Study the drawing (mm; zero at the part's minimum x, y, z) and answer. Give positions to 0.01 mm unless a question says otherwise; leave off trailing zeros. Write each loop counter-clockwise with the first axis right and the second up, starting at its lowest first coordinate (ties: lowest second). Pieces come first, ordered by that corner, then holes. Notation, with made-up numbers: (7, 18.5) - (22, 18.5) arc R12 cw to (22, 29.5) - close; hole circle Ø11 at (0, -3.5). An arc over 180 degrees is marked (long way). Answer in a Markdown table with one row per item. Add a question column.
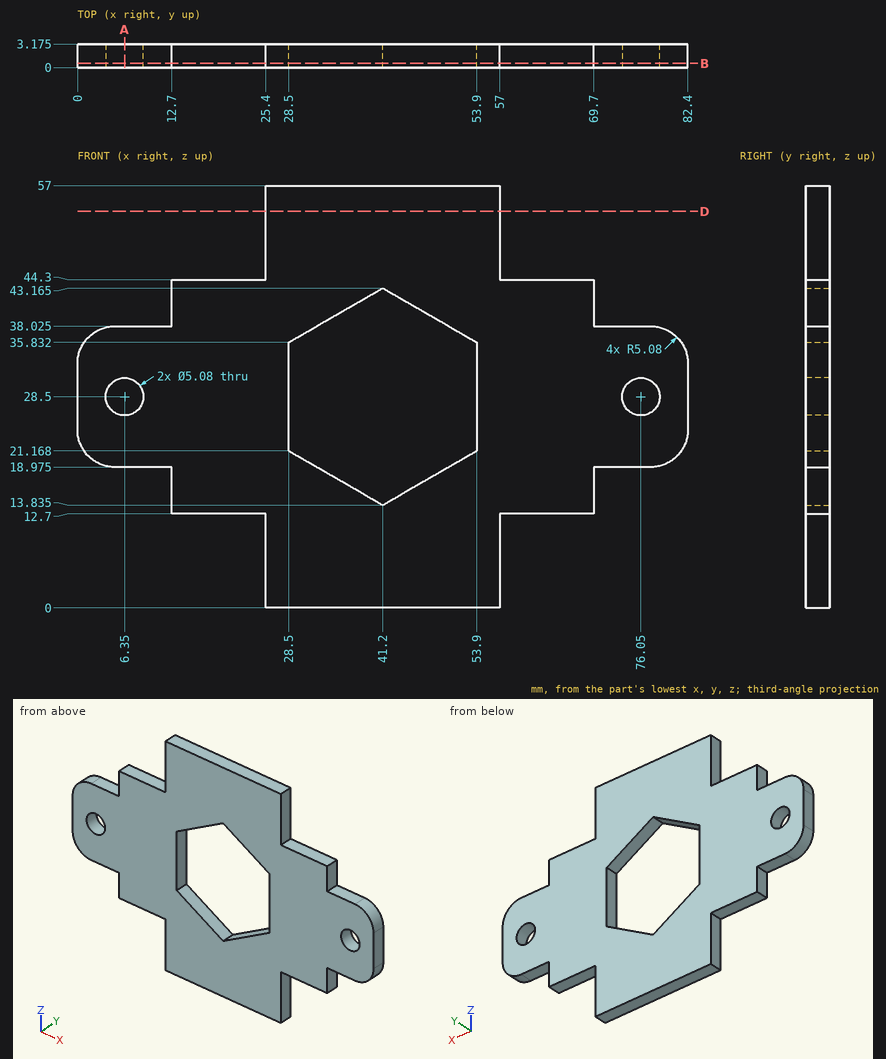
1. Section B-B (y = 0.55) is taken. State how many separate pieces and enclosed holes the cut face has, and give its area (3 significant figures).
2. Section D-D (z = 53.5) is taken. Give the vertices of the cut face in (x, y) (1 decimal), and give its area (3 significant figures).
3. Given pin 1 Ø1 at (x, y) = (66, 2.5) entering from +Z; pin 2 Ø1.6 at (y, z) = (2, 42.5) entering from -X; pin 3 Ø1 at (x, y) = (66, 2) entering from -Z, each flat-ended and moving along its own axis, determine where each tip first touches the part or whether it passes through.
4. Straight lines are drawn through the part: L1, parallel to Z at x = 6.35, y = 1 (1 decimal); L2, parallel to X at y = 1.5, z = 32; L3, parallel to X at y = 2.8, z = 10. For each, find the intervals that lie inside material, in ascending order. Write a range as [from, to].
5. Section A-A (x = 6.35) is taken. Give the vertices of the cut face in (y, z) (1 decimal).
Geometry check:
| question | item | result |
|---|---|---|
| 1 | separate pieces | 1 |
| 1 | enclosed holes | 3 |
| 1 | area | 2,470 mm² |
| 2 | outline | (25.4, 0) - (57, 0) - (57, 3.2) - (25.4, 3.2) - close |
| 2 | area | 100 mm² |
| 3 | pin 1 | z = 44.3 |
| 3 | pin 2 | x = 12.7 |
| 3 | pin 3 | z = 12.7 |
| 4 | L1 | [19, 26], [31, 38] |
| 4 | L2 | [0, 28.5], [53.9, 82.4] |
| 4 | L3 | [25.4, 57] |
| 5 | outline | (0, 19) - (3.2, 19) - (3.2, 26) - (0, 26) - close; (0, 31) - (3.2, 31) - (3.2, 38) - (0, 38) - close |
